Could you check a few things on this model? Use its own coordinates, in mm. Face numbers are marked on the shaded views. A direction names the side the tool comes from. Coordinates: 2 decimals unless noted, no trailing zeros. Loops run counter-clockwise (first coordinate to the right, second up) from the corner with the lowest first, then second, coordinate; pieces in that order, holes last. Notation, with made-up numbers: (-16, 77) - (-2, 77) arc R19 ccw to (-2, 81) - close; hole circle Ø11 at (11, 38). An arc over 180 degrees is marked (long way). One line per question, with ' | ' between items. Start each with the question number.
1. We'd pull the mould along Z, two halves only. Please class the marked faces 6, 7 and 8: pulls with the +Z half, pulls with the -Z half, needs draft (parallel to the pull), parting line crosses it, or undercut.
2. Please list where these lines run through material, in increasing order: L1, parallel to Z at x = 0, y = -3.25; L2, parallel to Y at x = -2.75, z = 9.25; L3, parallel to Z at x = -6, y = -1. Write a range as [from, to].
3. I want a section at A-A, the plane z = 12.75. Write out the boundary of the cut face in (x, y), then the cut area to 3 significant figures.
4. Which directions (+Z, -Z, +X, -X, +Y, -Y) give clear straight access to the entire face, cutting with the end or side of a thin tool? Please do the marked faces 1, 2, 3, 4 and 5.
5. I'm going to push flat-ended pins straight in: P1, Ø3, axis at y = -9.5, z = 7.5, coming from the +X side; P2, Ø8, axis at x = 1, y = -22, coming from the -Z side; P3, Ø4, axis at x = 3.5, z = 10, coming from the -Y side. Where does each tip first touch, or does it pass through?
6. I want a section at B-B, the plane x = -2.5. Count the separate pieces of the cut face and the enclosed holes in it, then the cut area to 3 significant figures.
from build123d import *

# Parameters (mm, degrees)
SKETCH_3_R               = 3
CUT_EXTRUDE_1_DEPTH      = 19.2
EXTRUDE_1_DEPTH          = 6.75
EXTRUDE_1_DEPTH_BACK     = 6.75
SKETCH_5_R               = 3.2
CUT_EXTRUDE_2_DEPTH      = 6.75
CUT_EXTRUDE_2_DEPTH_BACK = 6.75
SKETCH_6_R               = 1.6
EXTRUDE_2_DEPTH          = 5
SKETCH_8_R               = 4
EXTRUDE_3_DEPTH          = 8
FILLET_1_R               = 1


with BuildPart() as part:
    # Sketch 1 → Revolve 1 (revolve)
    with BuildSketch(Plane(origin=(0, 0, 0), x_dir=(0, 0, -1), z_dir=(1, 0, 0)), mode=Mode.PRIVATE) as revolve_1_sk:
        with BuildLine():
            Line((-19.2, 0), (-19.2, 7.125))
            ThreePointArc((-19.2, 7.125), (-19.112132034, 7.337132034), (-18.9, 7.425))
            Line((-18.9, 7.425), (-18.24, 7.425))
            Line((-18.24, 7.425), (-18.24, 4.5))
            Line((-18.24, 4.5), (-17.76, 4.5))
            Line((-17.76, 4.5), (-17.76, 6.2125))
            ThreePointArc((-17.76, 6.2125), (-17.701421356, 6.353921356), (-17.56, 6.4125))
            Line((-17.56, 6.4125), (-16.8, 6.4125))
            Line((-16.8, 6.4125), (-15.6, 6.75))
            Line((-15.6, 6.75), (-7.68, 6.75))
            Line((-7.68, 6.75), (-6.46445454, 5.4))
            Line((-6.46445454, 5.4), (0, 5.4))
            ThreePointArc((0, 5.4), (3.818376618, 3.818376618), (5.4, 0))
            Line((5.4, 0), (-19.2, 0))
        make_face()
    revolve(revolve_1_sk.sketch.rotate(Axis((0, 0, -5.4), (0, 0, 1)), 270), axis=Axis((0, 0, -5.4), (0, 0, 1)))

    # Sketch 2 → Revolve 2 (revolve)
    with BuildSketch(Plane(origin=(0, 0, 0), x_dir=(0, 0, -1), z_dir=(1, 0, 0)), mode=Mode.PRIVATE) as revolve_2_sk:
        Polygon((-6.75, -14.728504785), (-6.75, -7.68), (-5.4, -6.46445454), (-5.4, 0), (0, 0), (0, -14.728504785), align=None)
    revolve(revolve_2_sk.sketch.rotate(Axis((0, 0, 0), (0, -1, 0)), 180), axis=Axis((0, 0, 0), (0, -1, 0)))

    # Sketch 3 → Cut-Extrude 1 (cut)
    with BuildSketch(Plane.XY):
        Circle(SKETCH_3_R)
    extrude(amount=CUT_EXTRUDE_1_DEPTH, mode=Mode.SUBTRACT)

    # Sketch 5 → Extrude 1 (add, two sides: drawn at the far end of the back side and taken through both)
    with BuildSketch(Plane(origin=(0, 0, 0), x_dir=(0, 0, -1), z_dir=(1, 0, 0)).offset(-EXTRUDE_1_DEPTH_BACK)):
        with Locations((-8, -8)):
            Circle(SKETCH_5_R)
    extrude(amount=EXTRUDE_1_DEPTH + EXTRUDE_1_DEPTH_BACK)

    # Sketch 6 → Cut-Extrude 2 (cut, two sides: drawn at the far end of the back side and taken through both)
    with BuildSketch(Plane(origin=(0, 0, 0), x_dir=(0, 0, -1), z_dir=(1, 0, 0)).offset(-CUT_EXTRUDE_2_DEPTH_BACK)):
        with Locations((-8, -8)):
            Circle(SKETCH_6_R)
    extrude(amount=CUT_EXTRUDE_2_DEPTH + CUT_EXTRUDE_2_DEPTH_BACK, mode=Mode.SUBTRACT)

    # Sketch 4 → Cut-Revolve 1 (revolve, cut)
    with BuildSketch(Plane(origin=(0, 0, 0), x_dir=(0, 0, -1), z_dir=(1, 0, 0)), mode=Mode.PRIVATE) as cut_revolve_1_sk:
        with BuildLine():
            Line((3, 0), (3, -39.2))
            Line((3, -39.2), (0, -39.2))
            Line((0, -39.2), (0, 3))
            ThreePointArc((0, 3), (2.121320344, 2.121320344), (3, 0))
        make_face()
    revolve(cut_revolve_1_sk.sketch.rotate(Axis((0, -19.2, 0), (0, 1, 0)), 270), axis=Axis((0, -19.2, 0), (0, 1, 0)), mode=Mode.SUBTRACT)

    # Sketch 7 → Extrude 2 (add)
    with BuildSketch(Plane.XZ.offset(14.728504785)):
        Polygon((-5.644667133, -3.701382574), (0.383157772, -6.73911642), (6.027824905, -3.037733846), (5.644667133, 3.701382574), (-0.383157772, 6.73911642), (-6.027824905, 3.037733846), align=None)
    extrude(amount=EXTRUDE_2_DEPTH)

    # Sketch 8 → Extrude 3 (add)
    with BuildSketch(Plane.XZ.offset(19.728504785)):
        with Locations(Location((0, 0, 0), (0, 0, 270))):
            Circle(SKETCH_8_R)
    extrude(amount=EXTRUDE_3_DEPTH)

    # Fillet 1
    fillet_1_edges = [part.edges().sort_by_distance(p)[0] for p in [
        (0, -27.728504785, 4),
    ]]
    fillet(fillet_1_edges, radius=FILLET_1_R)


solid = part.part
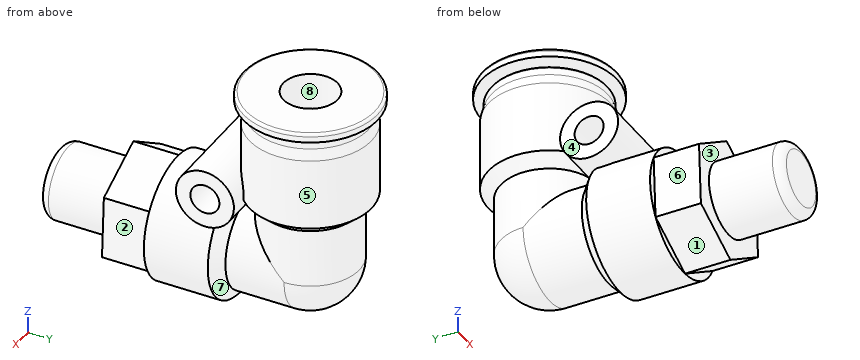
Results are:
1) face 6: pulls with the -Z half | face 7: undercut | face 8: needs draft
2) L1: z = [-5.4, -3], [3, 19.2] | L2: y = [-10.95, -9], [-7, -1.2], [1.2, 6.16] | L3: z = [7.08, 17.76], [18.24, 19.2]
3) outline: circle Ø13.5 at (0, 0); hole circle Ø6 at (0, 0) | area: 115 mm2
4) face 1: -Z, -X, -Y | face 2: +Z, +X, -Y | face 3: -Y | face 4: +Z, -Z, -X, +Y, -Y | face 5: none
5) P1: stops at x = 6.75 | P2: stops at z = -6.74 | P3: stops at y = -11.2
6) separate pieces: 1 | enclosed holes: 2 | area: 383 mm2
